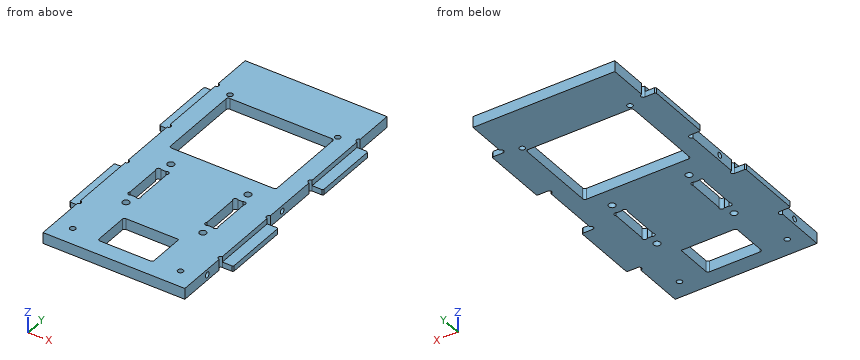
Autodesk Inventor part; units mm, degrees
ref_plane "YZ Plane" through (0, 0, 0) normal (1, 0, 0) x (0, 1, 0)
ref_plane "XZ Plane" through (0, 0, 0) normal (0, 1, 0) x (-1, 0, 0)
ref_plane "XY Plane" through (0, 0, 0) normal (0, 0, 1) x (1, 0, 0)
sketch "スケッチ1" plane through (0, 0, 0) normal (0, 0, 1) x (1, 0, 0)
  line L0 (-32.25, 65) -> (32.25, 65)
  line L1 (32.25, 65) -> (32.25, 47.1)
  line L2 (-32.25, -65) -> (-32.25, -47.1)
  line L3 (-32.25, 65) -> (32.25, -65) construction
  line L4 (32.25, 65) -> (-32.25, -65) construction
  line L5 (-32.25, 45) -> (-37.25, 45)
  line L6 (-37.25, 15) -> (-32.25, 15)
  line L7 (-37.25, 15) -> (-37.25, 45)
  line L8 (-32.25, -15) -> (-37.25, -15)
  line L9 (-37.25, -15) -> (-37.25, -45)
  line L10 (-37.25, -45) -> (-32.25, -45)
  arc A0 (-32.25, 45) -> (-32.25, 47.1) centre (-32.25, 46.05) ccw
  arc A1 (-32.25, 12.9) -> (-32.25, 15) centre (-32.25, 13.95) ccw
  arc A2 (-32.25, -15) -> (-32.25, -12.9) centre (-32.25, -13.95) ccw
  arc A3 (-32.25, -47.1) -> (-32.25, -45) centre (-32.25, -46.05) ccw
  line L11 (-32.25, 47.1) -> (-32.25, 65)
  line L12 (-32.25, 12.9) -> (-32.25, 15) construction
  line L13 (-32.25, -12.9) -> (-32.25, 12.9)
  line L14 (-32.25, -47.1) -> (-32.25, -45) construction
  line L15 (0, 65) -> (0, -65) construction
  arc A4 (32.25, -45) -> (32.25, -47.1) centre (32.25, -46.05) ccw
  line L16 (37.25, -45) -> (32.25, -45)
  line L17 (37.25, -15) -> (37.25, -45)
  line L18 (32.25, -15) -> (37.25, -15)
  arc A5 (32.25, -12.9) -> (32.25, -15) centre (32.25, -13.95) ccw
  arc A6 (32.25, 15) -> (32.25, 12.9) centre (32.25, 13.95) ccw
  line L19 (37.25, 15) -> (37.25, 45)
  line L20 (37.25, 15) -> (32.25, 15)
  line L21 (32.25, 45) -> (37.25, 45)
  arc A7 (32.25, 47.1) -> (32.25, 45) centre (32.25, 46.05) ccw
  line L22 (32.25, 47.1) -> (32.25, 45) construction
  line L23 (32.25, 12.9) -> (32.25, -12.9)
  line L24 (32.25, -47.1) -> (32.25, -65)
  line L25 (32.25, -12.9) -> (32.25, -15) construction
  line L26 (-32.25, -15) -> (-32.25, -12.9) construction
  line L27 (-32.25, -45) -> (-32.25, -15)
  line L28 (32.25, -15) -> (32.25, -45)
  line L29 (32.25, -45) -> (32.25, -47.1) construction
  line L30 (-20, -11.25) -> (-15, -11.25) construction
  line L31 (-15, -11.25) -> (-15, -31.25) construction
  line L32 (-15, -31.25) -> (-20, -31.25) construction
  line L33 (-20, -31.25) -> (-20, -11.25) construction
  line L34 (-20, -11.25) -> (-15, -31.25) construction
  line L35 (-15, -11.25) -> (-20, -31.25) construction
  line L36 (-20, 2.5) -> (-15, 2.5) construction
  line L37 (-15, 2.5) -> (-15, -45) construction
  line L38 (-15, -45) -> (-20, -45) construction
  line L39 (-20, -45) -> (-20, 2.5) construction
  line L40 (-20, 2.5) -> (-15, -45) construction
  line L41 (-15, 2.5) -> (-20, -45) construction
  circle A8 centre (-17.5, -36.25) radius 1.55
  line L42 (-20, -21.25) -> (-15, -21.25) construction
  line L43 (-17.5, 2.5) -> (-17.5, -45) construction
  circle A9 centre (-17.5, -6.25) radius 1.55
  circle A10 centre (17.5, -36.25) radius 1.55
  circle A11 centre (17.5, -6.25) radius 1.55
  line L44 (32.25, -65) -> (16.75, -65) construction
  line L45 (-12.5, -62.5) -> (-12.5, -45)
  line L46 (-12.5, -45) -> (0, -45)
  line L47 (12.5, -62.5) -> (12.5, -45)
  line L48 (12.5, -45) -> (0, -45)
  line L49 (-16.75, -65) -> (-32.25, -65) construction
  line L50 (16.75, -65) -> (-16.75, -65) construction
  line L51 (-32.25, 45) -> (-32.25, 47.1) construction
  line L52 (-32.25, 15) -> (-32.25, 45)
  line L53 (32.25, 15) -> (32.25, 12.9) construction
  line L54 (32.25, 45) -> (32.25, 15)
  circle A12 centre (-24.5, 43.5) radius 1.25
  line L55 (-32.25, 0) -> (32.25, 0) construction
  line L56 (-32.25, 46.5) -> (32.25, 46.5) construction
  circle A13 centre (-24.5, -61.5) radius 1.25
  circle A14 centre (24.5, 43.5) radius 1.25
  circle A15 centre (24.5, -61.5) radius 1.25
  circle A16 centre (-17.5, -36.25) radius 3 construction
  line L57 (-12.5, -62.5) -> (12.5, -62.5)
  line L58 (-24.25, 41.5) -> (24.25, 41.5)
  line L59 (24.25, 2.5) -> (-24.25, 2.5)
  line L60 (-24.25, 2.5) -> (-24.25, 41.5)
  line L61 (24.25, 2.5) -> (24.25, 41.5)
  line L62 (-20.05, -29.8151) -> (-18.5651, -31.3) construction
  line L63 (-19.3075, -30.5575) -> (-20.05, -31.3) construction
  arc A17 (-20.05, -29.8151) -> (-18.5651, -31.3) centre (-19.3075, -30.5575) ccw
  line L64 (-20.05, -11.2) -> (-18.5651, -11.2) construction
  line L65 (-14.95, -11.2) -> (-14.95, -12.6849) construction
  line L66 (-14.95, -31.3) -> (-16.4349, -31.3) construction
  line L67 (-20.05, -31.3) -> (-20.05, -29.8151) construction
  line L68 (-20.05, -11.2) -> (-14.95, -31.3) construction
  line L69 (-14.95, -11.2) -> (-20.05, -31.3) construction
  arc A18 (-16.4349, -31.3) -> (-14.95, -29.8151) centre (-15.6925, -30.5575) ccw
  arc A19 (-18.5651, -11.2) -> (-20.05, -12.6849) centre (-19.3075, -11.9425) ccw
  arc A20 (-14.95, -12.6849) -> (-16.4349, -11.2) centre (-15.6925, -11.9425) ccw
  line L70 (-20.05, -29.8151) -> (-20.05, -12.6849)
  line L71 (-18.5651, -31.3) -> (-20.05, -31.3) construction
  line L72 (-16.4349, -31.3) -> (-18.5651, -31.3)
  line L73 (-14.95, -29.8151) -> (-14.95, -31.3) construction
  line L74 (-20.05, -12.6849) -> (-20.05, -11.2) construction
  line L75 (-18.5651, -11.2) -> (-16.4349, -11.2)
  line L76 (-16.4349, -11.2) -> (-14.95, -11.2) construction
  line L77 (-14.95, -12.6849) -> (-14.95, -29.8151)
  arc A21 (18.5651, -31.3) -> (20.05, -29.8151) centre (19.3075, -30.5575) ccw
  arc A22 (14.95, -29.8151) -> (16.4349, -31.3) centre (15.6925, -30.5575) ccw
  arc A23 (16.4349, -11.2) -> (14.95, -12.6849) centre (15.6925, -11.9425) ccw
  arc A24 (20.05, -12.6849) -> (18.5651, -11.2) centre (19.3075, -11.9425) ccw
  line L78 (20.05, -29.8151) -> (20.05, -12.6849)
  line L79 (16.4349, -31.3) -> (18.5651, -31.3)
  line L80 (18.5651, -11.2) -> (16.4349, -11.2)
  line L81 (14.95, -12.6849) -> (14.95, -29.8151)
  line L82 (-32.25, -65) -> (-32.25, -70)
  line L83 (-32.25, -70) -> (32.25, -70)
  line L84 (32.25, -70) -> (32.25, -65)
  point P0 (0, 0)
  point P1 (0, 0)
  point P2 (0, 0)
  point P3 (28, 15)
  point P4 (28, 45)
  point P5 (-17.5, -21.25)
  point P6 (28, 45)
  point P7 (28, 15)
  dimension "d0" = 64.5
  dimension "d1" = 130
  dimension "d2" = 20
  dimension "d3" = 30
  dimension "d4" = 30
  dimension "d5" = 30
  dimension "d6" = 1.05
  dimension "d7" = 1.05
  dimension "d8" = 1.05
  dimension "d9" = 1.05
  dimension "d10" = 5
  dimension "d23" = 15
  dimension "d24" = 5
  dimension "d25" = 20
  dimension "d28" = 3.1
  dimension "d72" = 47.5
  dimension "d103" = 12.25
  dimension "d109" = 71.25
  dimension "d111" = 20
  dimension "d113" = 7.75
  dimension "d114" = 2.5
  dimension "d115" = 18.5
  dimension "d116" = 3
  dimension "d117" = 2.5
  dimension "d118" = 7.75
  dimension "d119" = 3.5
  dimension "d120" = 25
  dimension "d121" = 6
  dimension "d124" = 2.5
  dimension "d126" = 8
  dimension "d128" = 5
  dimension "d130" = 1.05
  dimension "d131" = 0.05
  dimension "d132" = 0.05
  dimension "d133" = 5
  dimension "d157" = 25
  dimension "d158" = 30
extrude "押し出し1" add sketch "スケッチ1" along normal blind 2.5
extrude "押し出し2" add sketch "スケッチ1" along normal blind 5 contours L0 L1 A7 L54 A6 L23 A5 L28 A4 L24 L84 L83 L82 L2 A3 L27 A2 L13 A1 L52 A0 L11
fillet "フィレット1" radius 1 7 edges at (-12.5, -45, 2.5) (-12.5, -62.5, 2.5) (12.5, -62.5, 2.5) (-24.25, 41.5, 2.5) (24.25, 41.5, 2.5) (24.25, 2.5, 2.5) (-24.25, 2.5, 2.5)
sketch "スケッチ7" plane through (32.25, -70, 0) normal (1, 0, 0) x (0, 0, -1)
  line L0 (0, 55) -> (-2.5, 55)
  line L1 (0, 57.1) -> (0, 82.9)
  line L2 (0, 0) -> (0, 22.9)
  point P0 (0, 70)
  point P1 (-2.5, 15)
  point P2 (-2.5, 65)
  point P3 (0, 25)
  dimension "d136" = 10
  dimension "d137" = 10
  dimension "d138" = 2.5
  dimension "d139" = 2.5
hole "穴6" at (32.25, -55, 2.5) at (32.25, -5, 2.5) direction (-1, 0, 0) diameter 2.459 depth 4
sketch "スケッチ8" plane through (-32.25, -70, 0) normal (-1, 0, 0) x (0, 0, 1)
  circle A0 centre (2.5, 15) radius 1.2295
  circle A1 centre (2.5, 65) radius 1.2295
  point P0 (0, 70)
  point P1 (2.5, 15)
  point P2 (2.5, 65)
hole "穴7" at (-32.25, -5, 2.5) at (-32.25, -55, 2.5) direction (1, 0, 0) diameter 2.459 depth 4
chamfer "面取り2" distance 0.5 angle 45 8 edges at (-37.25, -45, 1.25) (-37.25, -15, 1.25) (-37.25, 15, 1.25) (-37.25, 45, 1.25) (37.25, 15, 1.25) (37.25, 45, 1.25) (37.25, -15, 1.25) (37.25, -45, 1.25)
equation "\"d2\" = -0.5 * d4 + 0.5 * d1 - d3"
equation "\"d5\" = d3"
equation "\"d7\" = d6"
equation "\"d8\" = d7"
equation "\"d9\" = d8"
properties part number "Cockpit_horizontal_frame_02" material "アセタール樹脂、黒"
The listing builds one solid part. Answer for the finished solid, in the listing's coordinates (mm). Give positions to 0.01 mm unless a question says otherwise; leave off trailing zeros. Loops run counter-clockwise (first coordinate to the right, second up) from the corner with the lowest first, then second, coordinate; pieces in that order, holes last. Notation, with made-up numbers: (69, 30) - (77, 30) arc R14 ccw to (77, 43) - close; hole circle Ø7 at (49, 15.25). An arc over 180 degrees is marked (long way). Answer as a JSON object with one key per item and string values.
1. Find the intervals of material crossed by L1, parallel to Y at x = 6, z = 2; L2, parallel to Y at x = 17.5, z = 2.55; L3, parallel to X at y = -22.5, z = 1.3, in increasing order. Write a range as [from, to].
Determined:
{"L1": "[-70, -62.5], [-45, 2.5], [41.5, 65]", "L2": "[-70, -37.8], [-34.7, -31.3], [-11.2, -7.8], [-4.7, 2.5], [41.5, 65]", "L3": "[-37.25, -20.05], [-14.95, 14.95], [20.05, 37.25]"}
2. Flat-ended cylindrical pins translate along their axes: pin 1 Ø1.5 at (y, z) = (-54.5, 3.5) entering from +X; pin 2 Ø2 at (y, z) = (-54.5, 2.5) entering from -X; pin 3 Ø3 at (x, z) = (35.5, 1) entering from +Y. Find the tip coordinate at first contact, or state that the pin passes through.
Determined:
{"pin 1": "x = 32.25", "pin 2": "x = -32.25", "pin 3": "y = 45"}
3. A cutting plane is placed at A-A (x = 5). Write down the section's boundary in (y, z).
Determined:
{"outline": "(-70, 0) - (-62.5, 0) - (-62.5, 5) - (-70, 5) - close; (-45, 0) - (2.5, 0) - (2.5, 5) - (-45, 5) - close; (41.5, 0) - (65, 0) - (65, 5) - (41.5, 5) - close"}
4. A cutting plane is placed at B-B (y = 50.5). Write down the section's boundary in (x, z), then the cut area to 4 significant figures.
Determined:
{"outline": "(-32.25, 0) - (32.25, 0) - (32.25, 5) - (-32.25, 5) - close", "area": "322.5 mm²"}
